Geometry: final body of the model. Coordinates: model frame, mm. A direction names the side the tool comes from. Give positions to 0.01 mm unless a question says otherwise; leave off trailing zeros. Order: outer loops, then holes, each group sorted by start corner. A loop starts at its lowest first (then second) coordinate and runs counter-clockwise, first axis right, second up. Notation, with made-up numbers: M -33,-5 L -3,-5 A18 ccw -3,2 Z; hole C 85,-14 d6. An arc over 180 degrees is marked long. Use CSV: the item, a comma, the result in double quotes.
```python
from build123d import *

# Parameters (mm, degrees)
F0_R     = 90
F0_R_2   = 7
F1_DEPTH = 1
F2_R     = 8
F2_R_2   = 7
F3_DEPTH = 8
F4_R     = 90
F4_R_2   = 8
F4_R_3   = 7
F5_DEPTH = 1


with BuildPart() as f1:
    # F0 (on Right) → F1 (new body)
    with BuildSketch(Plane.YZ):
        Circle(F0_R)
        Circle(F0_R_2, mode=Mode.SUBTRACT)
    extrude(amount=F1_DEPTH)

    # F2 (on face) → F3 (join)
    with BuildSketch(Plane.YZ.offset(1)):
        Circle(F2_R)
        Circle(F2_R_2, mode=Mode.SUBTRACT)
    extrude(amount=F3_DEPTH)

    # F4 (on face) → F5 (join)
    with BuildSketch(Plane.YZ.offset(9)):
        Circle(F4_R)
        Circle(F4_R_2, mode=Mode.SUBTRACT)
        Circle(F4_R_2)
        Circle(F4_R_3, mode=Mode.SUBTRACT)
    extrude(amount=F5_DEPTH)


solid = f1.part
```
1. Section C-C, the plane y = -54.5. Return the cut outline in (x, z).
Answer:
outline,"M 0,-71.62 L 1,-71.62 L 1,71.62 L 0,71.62 Z; M 9,-71.62 L 10,-71.62 L 10,71.62 L 9,71.62 Z"
2. Reachability of faces 4 (the face through (0.493, 41.53, -79.845)), 5 (the face through (4.94, -1.73, -7.81)) from +Z, -Z, +X, -X, +Y, -Y: full face, straight path, thin tool, end or side. Return the list, or none.
Answer:
face 4,"+X, -X"
face 5,"none"
3. Section D-D, the plane x = 7.25. Return the cut outline in (y, z), plus the area to 3 significant figures.
Answer:
outline,"C 0,0 d16; hole C 0,0 d14"
area,"47.1 mm2"
4. Pull-direction query (X, two-part tool) for faces 1 (the face through (1, -1, -19)), 2 (the face through (9.493, 41.53, -79.845)), 3 (the face through (10, -1, -19)); classes: +X half, -X half, draft (parallel to the pull), parting line (faces both ways), or undercut.
Answer:
face 1,"undercut"
face 2,"draft"
face 3,"+X half"
5. Line query: line 1 (Z direction, x = 8, y = 0); line 2 (X direction, y = -55.5, z = 37.5). Output: solid intervals per line, ascending.
Answer:
line 1,"-8 to -7, 7 to 8"
line 2,"0 to 1, 9 to 10"
6. Pin query (flat end, axial travel): pin 1 Ø1.5 at (x, y) = (5, 6) entering from +Z; pin 2 Ø1.5 at (x, z) = (1, 38.5) entering from +Y; pin 3 Ø10 at (y, z) = (46, -6) entering from -X; pin 4 Ø5 at (x, y) = (3, 10) entering from -Z. Return the tip coordinate at first contact, or that it passes through.
Answer:
pin 1,"z = 6.04"
pin 2,"y = 81.7"
pin 3,"x = 0"
pin 4,"z = -89.6"
7. Section A-A, the plane y = 0. Return the cut outline in (x, z), plus the area to 3 significant figures.
Answer:
outline,"M 0,-90 L 1,-90 L 1,-8 L 9,-8 L 9,-90 L 10,-90 L 10,-7 L 0,-7 Z; M 0,7 L 10,7 L 10,90 L 9,90 L 9,8 L 1,8 L 1,90 L 0,90 Z"
area,"348 mm2"
